Design review of the part shown in the three views and the two pictorial views. Dimensions are in mm from the part's minimum x, y and z. A direction names the side the tool comes from. Round coordinates to 2 decimals unless told otherwise and drop trailing zeros. Loops run counter-clockwise (first coordinate to the right, second up) from the corner with the lowest first, then second, coordinate; pieces in that order, holes last. Notation, with made-up numbers: (-24.75, -36.75) -> (13.25, -36.75) arc R12 cw to (13.25, -26.75) -> close; hole circle Ø6 at (-28, 67.5). An arc over 180 degrees is marked (long way). Write each question's results on one line, items separated by ' | '. Start each with the question number.
Item 1: Mouldability with a two-part tool opening along X and no side actions: class the marked faces 1, 2 and 3 as pulls with the +X half, pulls with the -X half, needs draft (parallel to the pull), parting line crosses it, or undercut.
Item 2: We need section D-D (y = 3.5). Give the boundary of the cut face in (x, z), and give its area (3 significant figures).
Item 3: Clearance check with flat-ended pins moving along their axes: pin 1 Ø6 at (y, z) = (19, 8) entering from -X; pin 2 Ø5.5 at (x, z) = (20, 3.5) entering from -Y; pin 3 Ø5.5 at (y, z) = (19, 1.5) entering from +X; pin 4 Ø2.5 at (x, y) = (20, 36.5) entering from -Z. State where each tip first meets the part, or that it passes through.
Item 4: We need section A-A (y = 20). Give the boundary of the cut face in (x, z).
Item 5: We need section B-B (z = 1). Give the boundary of the cut face in (x, y).
Item 6: For L1, parallel to Y at x = 20, z = 7.7; L2, parallel to Y at x = 20, z = 1; L3, parallel to Z at x = 15, y = 3, list the stretches that pass through material, from the lowest coordinate up. Write a range as from..to.
Item 7: We need section C-C (x = 4.5). Give the boundary of the cut face in (y, z).
Item 8: Tool access review of the marked faces 4 and 5: name each direction out of +Z, -Z, +X, -X, +Y, -Y from which nothing blocks a thin tool from reaching the whole face with its end or side.
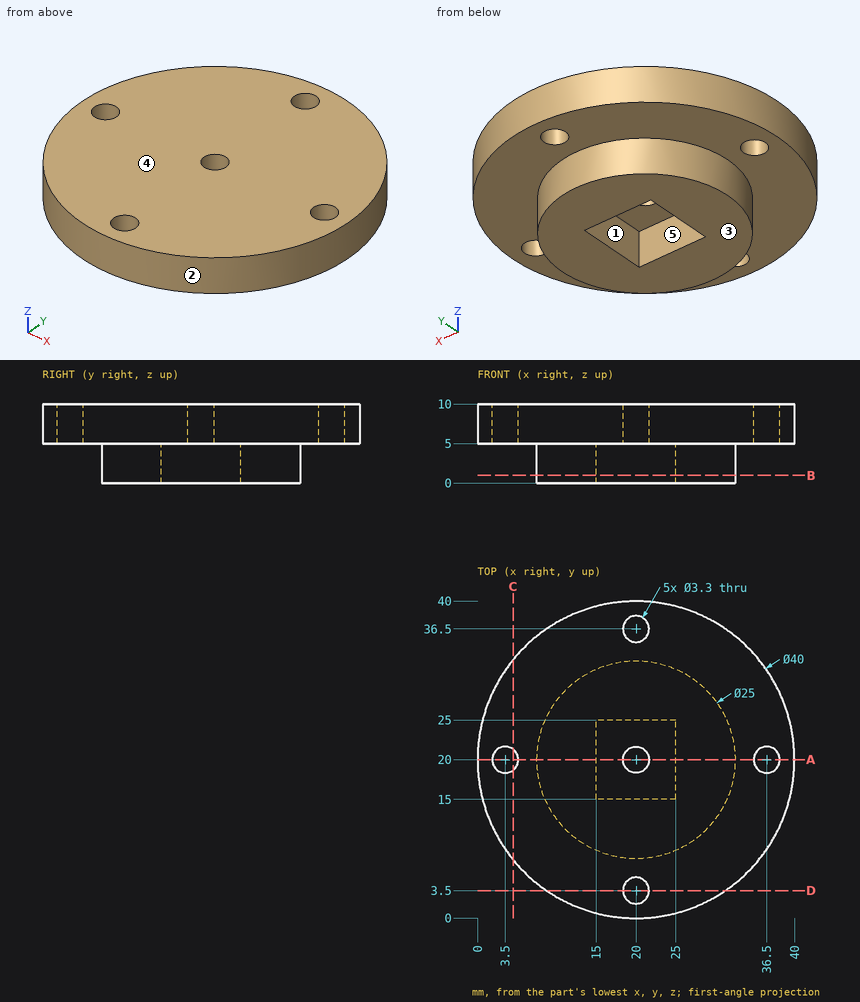
Here are the results:
1) face 1: undercut | face 2: parting line crosses it | face 3: needs draft
2) outline: (8.7, 5) -> (18.35, 5) -> (18.35, 10) -> (8.7, 10) -> close; (21.65, 5) -> (31.3, 5) -> (31.3, 10) -> (21.65, 10) -> close | area: 96.5 mm2
3) pin 1: stops at x = 0 | pin 2: stops at y = 0 | pin 3: stops at x = 32.5 | pin 4: passes through
4) outline: (0, 5) -> (1.85, 5) -> (1.85, 10) -> (0, 10) -> close; (5.15, 5) -> (7.5, 5) -> (7.5, 0) -> (15, 0) -> (15, 5) -> (18.35, 5) -> (18.35, 10) -> (5.15, 10) -> close; (21.65, 5) -> (25, 5) -> (25, 0) -> (32.5, 0) -> (32.5, 5) -> (34.85, 5) -> (34.85, 10) -> (21.65, 10) -> close; (38.15, 5) -> (40, 5) -> (40, 10) -> (38.15, 10) -> close
5) outline: circle Ø25 at (20, 20); hole (15, 15) -> (25, 15) -> (25, 25) -> (15, 25) -> close
6) L1: y = 0..1.85, 5.15..18.35, 21.65..34.85, 38.15..40 | L2: y = 7.5..15, 25..32.5 | L3: z = 5..10
7) outline: (7.36, 5) -> (18.69, 5) -> (18.69, 10) -> (7.36, 10) -> close; (21.31, 5) -> (32.64, 5) -> (32.64, 10) -> (21.31, 10) -> close
8) face 4: +Z, +X, -X, +Y, -Y | face 5: -Z
